from build123d import *

# Parameters (mm, degrees)
F0_R     = 42.5
F1_DEPTH = 195
F2_R     = 20.142482
F3_DEPTH = 30
F4_R     = 10
F5_R     = 6
F6_DEPTH = 16
F7_R     = 2


with BuildPart() as f1:
    # F0 (on Top) → F1 (new body)
    with BuildSketch(Plane.XY):
        Circle(F0_R)
    extrude(amount=F1_DEPTH)

    # F2 (on face) → F3 (join)
    with BuildSketch(Plane.XY.offset(195)):
        Circle(F2_R)
    extrude(amount=F3_DEPTH)

    # F4
    f4_edges = [f1.edges().sort_by_distance(p)[0] for p in [
        (-20.142482, 0, 225),
    ]]
    fillet(f4_edges, radius=F4_R)

    # F5 (on face) → F6 (join)
    with BuildSketch(Plane(origin=(0, 0, 0), x_dir=(1, 0, 0), z_dir=(0, 0, -1))):
        Circle(F5_R)
    extrude(amount=F6_DEPTH)

    # F7
    f7_edges = [f1.edges().sort_by_distance(p)[0] for p in [
        (-42.5, 0, 195),
        (-42.5, 0, 0),
    ]]
    fillet(f7_edges, radius=F7_R)


solid = f1.part
Source: CAD feature listing. Evaluate the final solid. Frame: model axes, mm. A direction names the side the tool comes from. Round coordinates to 2 decimals unless told otherwise and drop trailing zeros. Loops run counter-clockwise (first coordinate to the right, second up) from the corner with the lowest first, then second, coordinate; pieces in that order, holes last.
Q1. First-contact query: P1, Ø5, axis at x = -21, z = 121, coming from the +Y side; P2, Ø10, axis at y = -12, z = 136, coming from the +X side; P3, Ø2, axis at y = -20.5, z = 170, coming from the -X side. Flat tips, straight axial feed; report the tip coordinate or a pass-through.
Q2. Section A-A, the plane x = 0. Return loops of the section in (y, z), plus the area to 3 significant figures.
Q3. Ray query, line 1 (Z direction, x = -31, y = -15.5); line 2 (Y direction, x = -1, z = 193); line 3 (Z direction, x = -7.5, y = -4). Return the intervals inside material, ascending.
Q4. Access query for faces 1 (the face through (0, 0, 225)), 2 (the face through (-6, 0, -8)), 3 (the face through (-19, -8, 195)). Directions: +Z, -Z, +X, -X, +Y, -Y. A direction counts if a zero-diameter tool reaches every point of the face in a straight line with its end or side. Return the directions, or none.
Q5. Section C-C, the plane z = 88.5. Return loops of the section in (x, y), plus the area to 3 significant figures.
Solutions:
1. P1: stops at y = 38.26
1. P2: stops at x = 41.92
1. P3: stops at x = -37.76
2. outline: (-42.5, 2) arc R2 ccw to (-40.5, 0) - (-6, 0) - (-6, -16) - (6, -16) - (6, 0) - (40.5, 0) arc R2 ccw to (42.5, 2) - (42.5, 193) arc R2 ccw to (40.5, 195) - (20.14, 195) - (20.14, 215) arc R10 ccw to (10.14, 225) - (-10.14, 225) arc R10 ccw to (-20.14, 215) - (-20.14, 195) - (-40.5, 195) arc R2 ccw to (-42.5, 193) - close
2. area: 17,900 mm2
3. line 1: z = 0 to 195
3. line 2: y = -42.49 to 42.49
3. line 3: z = 0 to 225
4. face 1: +Z, +X, -X, +Y, -Y
4. face 2: -Z
4. face 3: +Z
5. outline: circle Ø85 at (0, 0)
5. area: 5,670 mm2
